Read the model definition and answer for the solid it produces. Units are mm, in the model's axes. A direction names the side the tool comes from. Round coordinates to 2 decimals unless told otherwise and drop trailing zeros. Order: outer loops, then holes, each group sorted by start corner. A loop starts at its lowest first (then second) coordinate and runs counter-clockwise, first axis right, second up. Notation, with made-up numbers: (-4, 85.25) - (48, 85.25) arc R14 cw to (48, 103.25) - close; hole circle Ø1 at (76.5, -6). An arc over 180 degrees is marked (long way). Put each result on its own line as item: value. Start each with the question number.
Q1. Section D-D on x = 5.75 is taken. Give the vertices of the cut face in (y, z).
Q2. Section A-A on y = 20.5 is taken. Give the vertices of the cut face in (x, z).
Q3. Which of the six approach directions +Z, -Z, +X, -X, +Y, -Y give full straight-line access (tool end or side, diameter ignored) to faces 1 (the face through (12.25, 17, 10)), 2 (the face through (23, 2, 10)), 3 (the face through (27.965, 4.699, 7.591)), 4 (the face through (4.949, 22.215, 8.93))?
Q4. Section B-B on x = 26.25 is taken. Give the vertices of the cut face in (y, z), then the cut area to 3 significant figures.
Q5. Section C-C on z = 12 is taken. Give the vertices of the cut face in (x, y).
Q6. Each of these flat-tipped pins is pushed along its axis until it touches: pin 1 Ø6 at (x, y) = (8, 6) entering from +Z; pin 2 Ø2 at (x, z) = (7, 7) entering from -Y; pin 3 Ø2.5 at (y, z) = (13, 10) entering from +X; pin 4 Ø3 at (x, y) = (23, 16.5) entering from -Z. Where does it stop, or does it pass through?
Q7. Find the intervals of material crossed by line 1 along Z through (x, y) = (22.5, 3.75); line 2 along Y through (x, z) = (19.5, 12.5); line 3 along X through (y, z) = (2.5, 12.5), in increasing order. Write a range as from..to.
Q8. For a pull along Y with two mould halves and no side action, classify faces 5 (the face through (15.969, 0.285, 0.301)), 6 (the face through (20.152, 22.215, 14.699)), 7 (the face through (21, 5, 7)) as pulls with the +Y half, pulls with the -Y half, needs draft (parallel to the pull), parting line crosses it, or undercut.
from build123d import *

# Parameters (mm, degrees)
PAD_DEPTH       = 15
SKETCH001_W     = 7
SKETCH001_H     = 22.5
POCKET_DEPTH    = 10
SKETCH003_W     = 3
SKETCH003_H     = 5
POCKET001_DEPTH = 22.501
FILLET_R        = 5
FILLET001_R     = 1
FILLET002_R     = 0.5


with BuildPart() as part:
    # Sketch → Pad (new body)
    with BuildSketch(Plane.XY):
        with BuildLine():
            ThreePointArc((18.25, 17.5), (12, 11.25), (18.25, 5))
            Line((28.25, 5), (18.25, 5))
            Line((28.25, 0), (28.25, 5))
            Line((0, 0), (28.25, 0))
            Line((0, 22.5), (0, 0))
            Line((28.25, 22.5), (0, 22.5))
            Line((28.25, 17.5), (28.25, 22.5))
            Line((18.25, 17.5), (28.25, 17.5))
        make_face()
    extrude(amount=PAD_DEPTH)

    # Sketch001 (on Face10 of Pad) → Pocket (cut)
    with BuildSketch(Plane.XY.offset(15)):
        with Locations((8.75, 11.25)):
            Rectangle(SKETCH001_W, SKETCH001_H)
    extrude(amount=-POCKET_DEPTH, mode=Mode.SUBTRACT)

    # Sketch003 → Pocket001 (cut, through all)
    with BuildSketch(Plane.XZ):
        with Locations((23.5, 7.5)):
            Rectangle(SKETCH003_W, SKETCH003_H)
    extrude(amount=-POCKET001_DEPTH, mode=Mode.SUBTRACT)

    # Fillet
    fillet_edges = [part.edges().sort_by_distance(p)[0] for p in [
        (0, 11.25, 0),
    ]]
    fillet(fillet_edges, radius=FILLET_R)

    # Fillet001
    fillet001_edges = [part.edges().sort_by_distance(p)[0] for p in [
        (0, 11.25, 15),
        (5.25, 11.25, 15),
        (2.625, 0, 15),
        (0, 0, 10),
        (0, 22.5, 10),
        (2.625, 22.5, 15),
        (20.25, 22.5, 15),
        (28.25, 20, 15),
        (23.25, 17.5, 15),
        (14.5, 16.25, 15),
        (12.25, 17.75, 15),
        (12.25, 4.75, 15),
        (23.25, 5, 15),
        (14.5, 6.25, 15),
        (28.25, 2.5, 15),
        (20.25, 0, 15),
        (28.25, 0, 7.5),
        (16.625, 0, 0),
        (1.464466, 0, 1.464466),
        (5.25, 0, 10),
        (8.75, 0, 5),
        (12.25, 0, 10),
        (12.25, 22.5, 10),
        (5.25, 22.5, 10),
        (8.75, 22.5, 5),
        (16.625, 22.5, 0),
        (1.464466, 22.5, 1.464466),
        (28.25, 5, 7.5),
        (28.25, 2.5, 0),
        (23.25, 5, 0),
        (12, 11.25, 0),
        (28.25, 17.5, 7.5),
        (28.25, 20, 0),
        (28.25, 22.5, 7.5),
        (23.25, 17.5, 0),
    ]]
    fillet(fillet001_edges, radius=FILLET001_R)

    # Fillet002
    fillet002_edges = [part.edges().sort_by_distance(p)[0] for p in [
        (25, 0, 7.5),
        (23.5, 0, 5),
        (22, 0, 7.5),
        (23.5, 0, 10),
        (23.5, 17.5, 10),
        (25, 17.5, 7.5),
        (23.5, 17.5, 5),
        (22, 17.5, 7.5),
        (25, 5, 7.5),
        (23.5, 5, 10),
        (22, 5, 7.5),
        (23.5, 5, 5),
        (23.5, 22.5, 10),
        (22, 22.5, 7.5),
        (23.5, 22.5, 5),
        (25, 22.5, 7.5),
    ]]
    fillet(fillet002_edges, radius=FILLET002_R)


solid = part.part
Findings:
1. outline: (0, 1) arc R1 ccw to (1, 0) - (21.5, 0) arc R1 ccw to (22.5, 1) - (22.5, 4) arc R1 ccw to (21.5, 5) - (1, 5) arc R1 ccw to (0, 4) - close
2. outline: (0, 5) arc R5 ccw to (5, 0) - (27.25, 0) arc R1 ccw to (28.25, 1) - (28.25, 14) arc R1 ccw to (27.25, 15) - (13.25, 15) arc R1 ccw to (12.25, 14) - (12.25, 5) - (5.25, 5) - (5.25, 14) arc R1 ccw to (4.25, 15) - (1, 15) arc R1 ccw to (0, 14) - close; hole (22, 5) - (25, 5) - (25, 10) - (22, 10) - close
3. face 1: +Z, +Y, -Y
3. face 2: +Y, -Y
3. face 3: +Z, -Z, +X
3. face 4: +Z, +Y
4. outline: (0, 1) arc R1 ccw to (1, 0) - (4, 0) arc R1 ccw to (5, 1) - (5, 14) arc R1 ccw to (4, 15) - (1, 15) arc R1 ccw to (0, 14) - close; (17.5, 1) arc R1 ccw to (18.5, 0) - (21.5, 0) arc R1 ccw to (22.5, 1) - (22.5, 14) arc R1 ccw to (21.5, 15) - (18.5, 15) arc R1 ccw to (17.5, 14) - close
4. area: 148 mm2
5. outline: (0, 1) arc R1 ccw to (1, 0) - (4.25, 0) arc R1 ccw to (5.25, 1) - (5.25, 21.5) arc R1 ccw to (4.25, 22.5) - (1, 22.5) arc R1 ccw to (0, 21.5) - close; (12.25, 1) arc R1 ccw to (13.25, 0) - (27.25, 0) arc R1 ccw to (28.25, 1) - (28.25, 4) arc R1 ccw to (27.25, 5) - (18.25, 5) arc R6.25 cw to (12.25, 9.5) - close; (12.25, 13) arc R6.25 cw to (18.25, 17.5) - (27.25, 17.5) arc R1 ccw to (28.25, 18.5) - (28.25, 21.5) arc R1 ccw to (27.25, 22.5) - (13.25, 22.5) arc R1 ccw to (12.25, 21.5) - close
6. pin 1: z = 14.66
6. pin 2: through
6. pin 3: x = 12.77
6. pin 4: z = 0.13
7. line 1: 0..5, 10..15
7. line 2: 0..5, 17.5..22.5
7. line 3: 0..5.25, 12.25..28.25
8. face 5: pulls with the -Y half
8. face 6: pulls with the +Y half
8. face 7: undercut
